Can you work these out from the model? Positions are in its coordinate system, mm. Face numbers are marked on the shaded views. A direction names the side the tool comes from. Coordinates: 2 decimals unless noted, no trailing zeros. Loops run counter-clockwise (first coordinate to the right, second up) from the corner with the lowest first, then second, coordinate; pieces in that order, holes last. Notation, with made-up numbers: M 17,30.25 L 35,30.25 A12 cw 35,34.25 Z; hole C -17.75,9 d9. An arc over 180 degrees is marked long. Return JSON: item names as keys, results as strings. Group by question number.
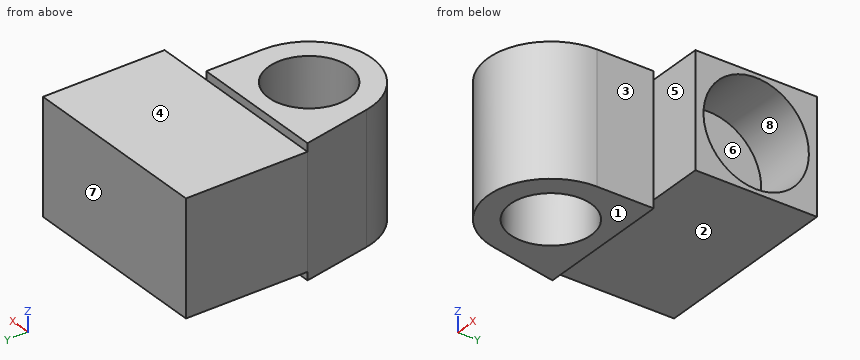
```python
from build123d import *

# Parameters (mm, degrees)
STOCK_4_1_START       = -70
STOCK_4_1_OUTLINE_R   = 50
STOCK_4_1_DEPTH       = 140
STOCK_4_1_START_2     = -80
STOCK_4_1_2_OUTLINE_R = 50
STOCK_4_1_2_DEPTH     = 160
SKETCH1_R             = 65
CUT_EXTRUDE1_DEPTH    = 80


# Read off the part's stored shape, not the designer's step: Stock-4-1
with BuildPart() as part:
    # Stock-4-1 outline → Stock-4-1 (new body)
    with BuildSketch(Plane.XY.offset(STOCK_4_1_START)):
        with BuildLine():
            Line((170.057165499, -75), (240, -75))
            Line((240, -75), (240, 75))
            Line((240, 75), (0, 75))
            Line((0, 75), (0, -75))
            Line((0, -75), (16.481058781, -159.787697142))
            ThreePointArc((16.481058781, -159.787697142), (99.985211319, -222.143205373), (170.057165499, -145))
            Line((170.057165499, -145), (170.057165499, -75))
        make_face()
        with Locations((92.557165499, -145)):
            Circle(STOCK_4_1_OUTLINE_R, mode=Mode.SUBTRACT)
    extrude(amount=STOCK_4_1_DEPTH)

    # Stock-4-1 2 outline → Stock-4-1 2 (add)
    with BuildSketch(Plane.XY.offset(STOCK_4_1_START_2)):
        with BuildLine():
            Line((170.057165499, -145), (170.057165499, -75))
            Line((170.057165499, -75), (0, -75))
            Line((0, -75), (16.481058781, -159.787697142))
            ThreePointArc((16.481058781, -159.787697142), (99.985211319, -222.143205373), (170.057165499, -145))
        make_face()
        with Locations((92.557165499, -145)):
            Circle(STOCK_4_1_2_OUTLINE_R, mode=Mode.SUBTRACT)
    extrude(amount=STOCK_4_1_2_DEPTH)

    # Sketch1 → Cut-Extrude1 (cut)
    with BuildSketch(Plane(origin=(240, 0, 0), x_dir=(0, 0, -1), z_dir=(1, 0, 0))):
        Circle(SKETCH1_R)
    extrude(amount=-CUT_EXTRUDE1_DEPTH, mode=Mode.SUBTRACT)


solid = part.part
```
1) If I drill on line 1 (Y direction, x = 211.5, z = 0); line 2 (Y direction, x = 229, z = -52); line 3 (X direction, y = -13.5, z = -41), over which ranges is the centre line in solid material (lowest first)? Write a range as from..to.
2) If we mould it in two halves opening along Y, with no side actions, what happens to the marked faces 5, 6, 7 and 8? For each: +Y half, -Y half, draft (parallel to the pull), parting line (faces both ways), or undercut.
3) Suppose I cut it at D-D, the plane x = 221. List the corners of the cut face in (y, z) for me.
4) For the marked faces 1, 2, 3 and 4, which set-ups out of +Z, -Z, +X, -X, +Y, -Y let a thin tool reach every point of the face, with its end or its side?
5) Suppose I cut it at B-B, the plane x = 55.5. List the corners of the cut face in (y, z) for me, then the cut area to 3 significant figures.
6) Suppose I cut it at A-A, the plane z = 0. List the corners of the cut face in (x, y) for me.
7) Suppose I cut it at C-C, the plane y = 0. List the corners of the cut face in (x, z) for me.
8) For pin 1 (10 mm diameter, centred on y = -154.5, z = 30, fed in from -X); pin 2 (12 mm diameter, centred on y = -121.5, z = 19, fed in from -X); pin 3 (3 mm diameter, centred on x = 123, z = -74, fed in from +Y), each with a flat end and sliding along its axis, tell me the tip position at first contact or that it passes through.
Returned:
{
 "1": {"line 1": "y = -75..-65, 65..75", "line 2": "y = -75..-39, 39..75", "line 3": "x = 0..160"},
 "2": {"face 5": "-Y half", "face 6": "undercut", "face 7": "+Y half", "face 8": "undercut"},
 "3": {"outline": "M -75,-70 L 75,-70 L 75,70 L -75,70 Z; hole C 0,0 d130"},
 "4": {"face 1": "-Z, +X, -X, +Y, -Y", "face 2": "-Z, +X, -X, +Y", "face 3": "+Z, -Z, +X, -Y", "face 4": "+Z, +X, -X, +Y"},
 "5": {"outline": "M -213.07,-80 L -178.57,-80 L -178.57,80 L -213.07,80 Z; M -111.43,-80 L -75,-80 L -75,-70 L 75,-70 L 75,70 L -75,70 L -75,80 L -111.43,80 Z", "area": "32,300 mm²"},
 "6": {"outline": "M 0,-75 L 16.48,-159.79 A77.5 ccw 170.06,-145 L 170.06,-75 L 240,-75 L 240,-65 L 160,-65 L 160,65 L 240,65 L 240,75 L 0,75 Z; hole C 92.56,-145 d100"},
 "7": {"outline": "M 0,-70 L 240,-70 L 240,-65 L 160,-65 L 160,65 L 240,65 L 240,70 L 0,70 Z"},
 "8": {"pin 1": "stops at x = 14.48", "pin 2": "stops at x = 7.87", "pin 3": "stops at y = -75"}
}
